Design review of the part built by this model. Coordinates are the model's own, in mm. Coordinates: 2 decimals unless noted, no trailing zeros. Loops run counter-clockwise (first coordinate to the right, second up) from the corner with the lowest first, then second, coordinate; pieces in that order, holes last. Notation, with made-up numbers: M 12,3.5 L 60,3.5 A31 ccw 60,40.5 Z; hole C 45.5,80 d4. An arc over 180 degrees is marked long. One line per item, written item: value.
```python
from build123d import *

# Parameters (mm, degrees)
F0_W     = 148.951292
F0_H     = 150.254234
F0_R     = 46.06604
F1_DEPTH = 100


with BuildPart() as f1:
    # F0 (on Top) → F1 (new body)
    with BuildSketch(Plane.XY):
        Rectangle(F0_W, F0_H)
        with Locations((1.823949, 0)):
            Circle(F0_R, mode=Mode.SUBTRACT)
        with Locations((-148.951292, 0)):
            Rectangle(F0_W, F0_H)
        with Locations((-150.775241, 0)):
            Circle(F0_R, mode=Mode.SUBTRACT)
    extrude(amount=F1_DEPTH)


solid = f1.part
```
(1) We need section A-A on y = 0. State the section outline as (x, z) points, then the cut area to 3 significant figures.
Reply:
outline: M -223.43,0 L -196.84,0 L -196.84,100 L -223.43,100 Z; M -104.71,0 L -44.24,0 L -44.24,100 L -104.71,100 Z; M 47.89,0 L 74.48,0 L 74.48,100 L 47.89,100 Z
area: 11,400 mm2
(2) We need section D-D on y = -28. State the section outline as (x, z) points.
Reply:
outline: M -223.43,0 L -187.36,0 L -187.36,100 L -223.43,100 Z; M -114.2,0 L -34.76,0 L -34.76,100 L -114.2,100 Z; M 38.4,0 L 74.48,0 L 74.48,100 L 38.4,100 Z
(3) Mouldability with a two-part tool opening along X and no side actions: class faces 1 (the cylindrical face through (-187.33, -28.03, 49.3)), 2 (the flat face through (-223.427, -1, 49)), 3 (the flat face through (-77, 1, 0)) as released by +X, released by -X, zero draft, split by the parting line, or undercut.
Reply:
face 1: undercut
face 2: released by -X
face 3: zero draft
(4) We need section C-C on z = 27.5. State the section outline as (x, y) points, then the cut area to 3 significant figures.
Reply:
outline: M -223.43,-75.13 L 74.48,-75.13 L 74.48,75.13 L -223.43,75.13 Z; hole C -150.78,0 d92.13; hole C 1.82,0 d92.13
area: 31,400 mm2
(5) We need section B-B on x = -117. State the section outline as (y, z) points.
Reply:
outline: M -75.13,0 L -31.33,0 L -31.33,100 L -75.13,100 Z; M 31.33,0 L 75.13,0 L 75.13,100 L 31.33,100 Z
(6) To check wall thickness, follow line 1 along X through (y, z) = (7.5, 68); line 2 along X through (y, z) = (11, 86.5); line 3 along Y through (x, z) = (-114, 71.5). State the ranges of each line that lie inside material, in increasing order. Write a range as [from, to].
Reply:
line 1: x = [-223.43, -196.23], [-105.32, -43.63], [47.28, 74.48]
line 2: x = [-223.43, -195.51], [-106.04, -42.91], [46.56, 74.48]
line 3: y = [-75.13, -27.74], [27.74, 75.13]
(7) Insertion check: pin 1 (8 mm diameter, centred on x = -66.5, y = 22, fed in from -Z); pin 2 (12 mm diameter, centred on x = 13, y = 33.5, fed in from -Z) (3 decimals). Each pin has a flat end and moves straight along its axis. Give the tip position at first contact, or say it passes through.
Reply:
pin 1: stops at z = 0
pin 2: passes through
